Can you work these out from the model? Positions are in its coordinate system, mm. A direction names the side the tool comes from. Give positions to 0.01 mm unless a question says otherwise; leave off trailing zeros. Order: outer loops, then holes, each group sorted by start corner. A loop starts at its lowest first (then second) coordinate and runs counter-clockwise, first axis right, second up. Notation, with made-up numbers: M 57.25,80 L 104.25,80 A29 ccw 104.25,100 Z; hole C 24,51.5 d5. An arc over 180 degrees is marked long. Write each question's results on one line, items separated by ' | '.
from build123d import *

# Parameters (mm, degrees)
SKETCH2_W                  = 50
SKETCH2_H                  = 50
BOSS_EXTRUDE1_DEPTH        = 6
SKETCH3_W                  = 50
SKETCH3_H                  = 19.118802154
BOSS_EXTRUDE2_DEPTH        = 9.5
BOSS_EXTRUDE3_DEPTH        = 12
SKETCH6_R                  = 3.6
SKETCH6_R_2                = 2.55
CUT_EXTRUDE2_DEPTH         = 41.193638748
SKETCH7_R                  = 5.05
SKETCH7_R_2                = 6
CUT_EXTRUDE3_DEPTH         = 2
M4X0_7_TAPPED_HOLE1_REACH  = 45.37
M4X0_7_TAPPED_HOLE1_BORE_R = 1.65
M4X0_7_TAPPED_HOLE2_D      = 3.3
M4X0_7_TAPPED_HOLE2_DEPTH  = 10
M4X0_7_TAPPED_HOLE2_TIP    = 0.991420021
FILLET1_R                  = 4.635
M3X0_5_TAPPED_HOLE1_D      = 2.5
M4X0_7_TAPPED_HOLE3_D      = 3.3
M4X0_7_TAPPED_HOLE3_DEPTH  = 6
M4X0_7_TAPPED_HOLE3_TIP    = 0.991420021
SKETCH17_R                 = 1.25
CUT_EXTRUDE4_DEPTH         = 60.080695659
SKETCH18_OUTSIDE_W         = 67.008
SKETCH18_OUTSIDE_H         = 67.008
SKETCH18_OUTSIDE_R         = 3
CUT_EXTRUDE5_DEPTH         = 2


with BuildPart() as part:
    # Sketch2 → Boss-Extrude1 (new body)
    with BuildSketch(Plane(origin=(0, 0, 0), x_dir=(0, 0, -1), z_dir=(1, 0, 0))):
        Rectangle(SKETCH2_W, SKETCH2_H)
    extrude(amount=BOSS_EXTRUDE1_DEPTH)

    # Sketch3 → Boss-Extrude2 (add, symmetric)
    with BuildSketch(Plane(origin=(25, 0, 0), x_dir=(0, 0, 1), z_dir=(0, 1, 0))):
        with Locations((0, -34.559401077)):
            Rectangle(SKETCH3_W, SKETCH3_H)
        with BuildLine():
            Line((-19, -32.42820323), (-19, -36.618802154))
            ThreePointArc((-19, -36.618802154), (-15, -40.618802154), (-11, -36.618802154))
            Line((-11, -36.618802154), (-11, -32.42820323))
            Line((-11, -32.42820323), (-11, -27.809401077))
            Line((-11, -27.809401077), (-15, -25.5))
            Line((-15, -25.5), (-19, -27.809401077))
            Line((-19, -27.809401077), (-19, -32.42820323))
        make_face(mode=Mode.SUBTRACT)
        with BuildLine():
            Line((11, -36.618802154), (11, -32.42820323))
            Line((11, -32.42820323), (11, -27.809401077))
            Line((11, -27.809401077), (15, -25.5))
            Line((15, -25.5), (19, -27.809401077))
            Line((19, -27.809401077), (19, -32.42820323))
            Line((19, -32.42820323), (19, -36.618802154))
            ThreePointArc((19, -36.618802154), (15, -40.618802154), (11, -36.618802154))
        make_face(mode=Mode.SUBTRACT)
    extrude(amount=BOSS_EXTRUDE2_DEPTH, both=True)

    # Sketch5 → Boss-Extrude3 (add)
    with BuildSketch(Plane(origin=(9.5, 9.5, 0), x_dir=(0, 0, 1), z_dir=(0, -1, 0))):
        Polygon((-19, 16), (-11, 16), (-11, 12.309401077), (-15, 10), (-19, 12.309401077), align=None)
        Polygon((11, 16), (19, 16), (19, 12.309401077), (15, 10), (11, 12.309401077), align=None)
    extrude(amount=BOSS_EXTRUDE3_DEPTH)

    # Sketch6 → Cut-Extrude2 (cut, through all)
    with BuildSketch(Plane(origin=(0, 0, 0), x_dir=(0, 0, -1), z_dir=(1, 0, 0))):
        with Locations((-15, 15.95)):
            Circle(SKETCH6_R)
        with Locations((15, 15.95)):
            Circle(SKETCH6_R)
        with Locations((-15, -15.95)):
            Circle(SKETCH6_R_2)
        with Locations((15, -15.95)):
            Circle(SKETCH6_R_2)
    extrude(amount=CUT_EXTRUDE2_DEPTH, mode=Mode.SUBTRACT)

    # Sketch7 → Cut-Extrude3 (cut)
    with BuildSketch(Plane.ZY):
        with Locations((-15, -15.95)):
            Circle(SKETCH7_R)
        with Locations((15, -15.95)):
            Circle(SKETCH7_R)
        with Locations((-15, 15.95)):
            Circle(SKETCH7_R_2)
        with Locations((15, 15.95)):
            Circle(SKETCH7_R_2)
    extrude(amount=-CUT_EXTRUDE3_DEPTH, mode=Mode.SUBTRACT)

    # M4x0.7 Tapped Hole1 bore → M4x0.7 Tapped Hole1 (cut, up to next)
    with BuildSketch(Plane(origin=(-19.118802154, 0, 0), x_dir=(0, -1, 0), z_dir=(-1, 0, 0)), mode=Mode.PRIVATE) as m4x0_7_tapped_hole1_sk1:
        with Locations((5.5, -15)):
            Circle(M4X0_7_TAPPED_HOLE1_BORE_R)
    m4x0_7_tapped_hole1_tool1 = extrude(m4x0_7_tapped_hole1_sk1.sketch, amount=-M4X0_7_TAPPED_HOLE1_REACH, mode=Mode.PRIVATE) & part.part
    # M4x0.7 Tapped Hole1 bore → M4x0.7 Tapped Hole1 (cut, up to next)
    with BuildSketch(Plane(origin=(-19.118802154, 0, 0), x_dir=(0, -1, 0), z_dir=(-1, 0, 0)), mode=Mode.PRIVATE) as m4x0_7_tapped_hole1_sk2:
        with Locations((5.5, 15)):
            Circle(M4X0_7_TAPPED_HOLE1_BORE_R)
    m4x0_7_tapped_hole1_tool2 = extrude(m4x0_7_tapped_hole1_sk2.sketch, amount=-M4X0_7_TAPPED_HOLE1_REACH, mode=Mode.PRIVATE) & part.part
    add(m4x0_7_tapped_hole1_tool1.solids().sort_by_distance((-19.118802, -5.5, -15))[0], mode=Mode.SUBTRACT)
    add(m4x0_7_tapped_hole1_tool2.solids().sort_by_distance((-19.118802, -5.5, 15))[0], mode=Mode.SUBTRACT)

    # M4x0.7 Tapped Hole2
    with Locations(Plane.ZY.offset(19.118802154)):
        with Locations((-9.525, 1.96821034), (9.525, 1.96821034)):
            Hole(M4X0_7_TAPPED_HOLE2_D / 2, depth=M4X0_7_TAPPED_HOLE2_DEPTH)
            with Locations((0, 0, -(M4X0_7_TAPPED_HOLE2_DEPTH + M4X0_7_TAPPED_HOLE2_TIP / 2))):  # 118° drill point
                Cone(0, M4X0_7_TAPPED_HOLE2_D / 2, M4X0_7_TAPPED_HOLE2_TIP, mode=Mode.SUBTRACT)

    # Fillet1
    fillet1_edges = [part.edges().sort_by_distance(p)[0] for p in [
        (3, -25, -25),
        (3, -25, 25),
        (3, 25, 25),
        (3, 25, -25),
    ]]
    fillet(fillet1_edges, radius=FILLET1_R)

    # M3x0.5 Tapped Hole1 (through all)
    with Locations(Plane.ZY):
        with Locations((0, 21.5), (0, -21.5), (0, -13.5), (0, 13.5)):
            Hole(M3X0_5_TAPPED_HOLE1_D / 2)

    # M4x0.7 Tapped Hole3
    with Locations(Plane(origin=(0, 9.5, 0), x_dir=(1, 0, 0), z_dir=(0, 1, 0))):
        with Locations((-4.95, 0)):
            Hole(M4X0_7_TAPPED_HOLE3_D / 2, depth=M4X0_7_TAPPED_HOLE3_DEPTH)
            with Locations((0, 0, -(M4X0_7_TAPPED_HOLE3_DEPTH + M4X0_7_TAPPED_HOLE3_TIP / 2))):  # 118° drill point
                Cone(0, M4X0_7_TAPPED_HOLE3_D / 2, M4X0_7_TAPPED_HOLE3_TIP, mode=Mode.SUBTRACT)

    # Sketch17 → Cut-Extrude4 (cut, through all)
    with BuildSketch(Plane(origin=(0, 0, -25), x_dir=(-1, 0, 0), z_dir=(0, 0, -1))):
        with Locations((3.3, 0)):
            Circle(SKETCH17_R)
    extrude(amount=-CUT_EXTRUDE4_DEPTH, mode=Mode.SUBTRACT)

    # Sketch18 outside → Cut-Extrude5 (cut)
    with BuildSketch(Plane.ZY.offset(19.118802154)):
        Rectangle(SKETCH18_OUTSIDE_W, SKETCH18_OUTSIDE_H)
        with Locations((-9.525, 1.96821034)):
            Circle(SKETCH18_OUTSIDE_R, mode=Mode.SUBTRACT)
        with Locations((9.525, 1.96821034)):
            Circle(SKETCH18_OUTSIDE_R, mode=Mode.SUBTRACT)
    extrude(amount=-CUT_EXTRUDE5_DEPTH, mode=Mode.SUBTRACT)


solid = part.part
(1) Imagine slicing it at D-D, the plane y = 13.5. Write out the boundary of the cut face in (x, z), plus the area to 3 significant figures.
Data:
outline: M 0,-25 L 6,-25 L 6,-17.64 L 2,-17.64 L 2,-20.48 L 0,-20.48 Z; M 0,-9.52 L 2,-9.52 L 2,-12.36 L 6,-12.36 L 6,-1.25 L 0,-1.25 Z; M 0,1.25 L 6,1.25 L 6,12.36 L 2,12.36 L 2,9.52 L 0,9.52 Z; M 0,20.48 L 2,20.48 L 2,17.64 L 6,17.64 L 6,25 L 0,25 Z | area: 199 mm2
(2) Imagine slicing it at C-C, the plane y = -5.5. Write out the boundary of the cut face in (x, z), plus the area to 3 significant figures.
Data:
outline: M -17.12,-25 L 6,-25 L 6,25 L -17.12,25 L -17.12,16.65 L -15.26,16.65 A4 cw -11.62,19 L -2.81,19 L -0.5,15 L -2.81,11 L -11.62,11 A4 cw -15.26,13.35 L -17.12,13.35 L -17.12,-13.35 L -15.26,-13.35 A4 cw -11.62,-11 L -2.81,-11 L -0.5,-15 L -2.81,-19 L -11.62,-19 A4 cw -15.26,-16.65 L -17.12,-16.65 Z | area: 936 mm2
(3) Imagine slicing it at A-A, the plane y = -15.95. Write out the boundary of the cut face in (x, z), plus the area to 3 significant figures.
Data:
outline: M 0,-25 L 6,-25 L 6,-17.55 L 2,-17.55 L 2,-20.05 L 0,-20.05 Z; M 0,-9.95 L 2,-9.95 L 2,-12.45 L 6,-12.45 L 6,12.45 L 2,12.45 L 2,9.95 L 0,9.95 Z; M 0,20.05 L 2,20.05 L 2,17.55 L 6,17.55 L 6,25 L 0,25 Z | area: 219 mm2
(4) Imagine slicing it at B-B, the plane x = 3.25. Count the separate pieces of the cut face and the enclosed holes in it, plus the area to 3 significant figures.
Data:
separate pieces: 1 | enclosed holes: 8 | area: 2,340 mm2
(5) I need wall thicknesses on L1, parallel to Y at x = 1.6, z = 15; L2, parallel to Y at x = 2.95, z = -15; L3, parallel to Z at x = 4.15, y = 15.95. Which ranges of each line are inside material? Lowest first, please. Write a range as from..to.
Data:
L1: y = -25..-21, -10.9..9.95, 21.95..25 | L2: y = -25..-18.5, -13.4..12.35, 19.55..25 | L3: z = -25..-18.6, -11.4..11.4, 18.6..25
(6) For faces 4 (the face through (-15.618, 0.133, 15.088)), 5 (the face through (-4, -2.5, 15)), 6 (the face through (-14.05, 1.34, 8)), 7 (the face through (-8, -9.5, 0)), 8 (the face through (-9, 9.5, 0)), which set-ups out of +Z, -Z, +X, -X, +Y, -Y let a thin tool reach every point of the face, with its end or its side?
Data:
face 4: +Y, -Y | face 5: -Y | face 6: -X | face 7: +Z, -Z, -X, -Y | face 8: +Z, -Z, -X, +Y
(7) Will these pins go through, and if not, where does the flat tip stop? P1, Ø3, axis at y = 1.97, z = -9.52, coming from the -X side; P2, Ø12.5, axis at y = 16, z = -1.5, coming from the -X side; P3, Ø14, axis at y = 15.95, z = -15, coming from the -X side; P4, Ø15.5, axis at y = 15.95, z = 15, coming from the +X side.
Data:
P1: stops at x = -9.03 | P2: stops at x = 0 | P3: stops at x = -17.12 | P4: stops at x = 6
(8) We'd pull the mould along Z, two halves only. Please class faces 1 (the face through (3.972, -17.502, 17.024)), 2 (the face through (-6, 0, -25)), 3 (the face through (-2.05, 0.05, -0.35)): +Z half, -Z half, draft (parallel to the pull), parting line (faces both ways), or undercut.
Data:
face 1: undercut | face 2: -Z half | face 3: draft
